For this review, take the finished solid that the model builds, in its own axes (mm). Face numbers are marked on the shaded views. A direction names the side the tool comes from. Round coordinates to 2 decimals unless told otherwise and drop trailing zeros. Loops run counter-clockwise (first coordinate to the right, second up) from the corner with the lowest first, then second, coordinate; pieces in that order, holes last.
1) Tool access review of the marked faces 1 and 2: name each direction out of +Z, -Z, +X, -X, +Y, -Y from which nothing blocks a thin tool from reaching the whole face with its end or side.
2) Wall thickness on L1, parallel to Z at x = 0, y = 0.3; L2, parallel to Y at x = 0, z = 50.7; L3, parallel to Y at x = 0, z = 51.45: over which ranges is each line inside the solid? List them lowest first.
3) Insertion check: pin 1 (4.5 mm diameter, centred on x = 0.5, z = 13.5, fed in from +Y); pin 2 (1 mm diameter, centred on x = 5.5, y = 45, fed in from -Z); pin 3 (4 mm diameter, centred on x = 0, z = 34.3, fed in from -Y). Each pin has a flat end and moves straight along its axis. Give the tip position at first contact, or say it passes through.
4) Take a section at B-B (x = 0). State the section outline as (y, z) points.
5) Take a section at D-D (x = 4.75). State the section outline as (y, z) points, then the cut area to 3 significant figures.
6) Take a section at A-A (y = 16.7). State the section outline as (x, z) points, then the cut area to 3 significant figures.
7) Take a section at C-C (z = 9.8). State the section outline as (x, y) points, then the cut area to 3 significant figures.
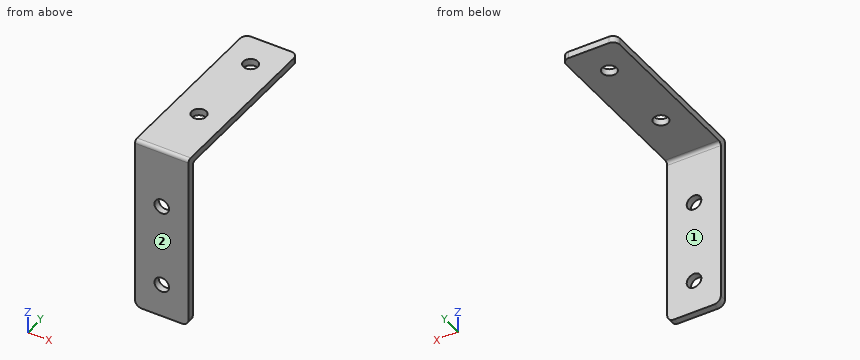
```python
from build123d import *

# Parameters (mm, degrees)
SKETCH_1_W          = 15.8
SKETCH_1_H          = 2
EXTRUDE_1_DEPTH     = 52
SKETCH_2_W          = 15.8
SKETCH_2_H          = 2
EXTRUDE_2_DEPTH     = 50
FILLET_5_R          = 1
FILLET_6_R          = 1
FILLET_7_R          = 2
FILLET_8_R          = 2
SKETCH_3_R          = 2.15
CUT_EXTRUDE_1_DEPTH = 50
SKETCH_8_R          = 2.15
CUT_EXTRUDE_3_DEPTH = 50


with BuildPart() as part:
    # 草圖1 → 填料-伸長1 (new body)
    with BuildSketch(Plane.XY):
        Rectangle(SKETCH_1_W, SKETCH_1_H)
    extrude(amount=EXTRUDE_1_DEPTH)

    # 草圖2 → 填料-伸長2 (add)
    with BuildSketch(Plane(origin=(0, 1, 0), x_dir=(1, 0, 0), z_dir=(0, 1, 0))):
        with Locations((0, -51)):
            Rectangle(SKETCH_2_W, SKETCH_2_H)
    extrude(amount=EXTRUDE_2_DEPTH)

    # 圓角5
    fillet_5_edges = [part.edges().sort_by_distance(p)[0] for p in [
        (0, -1, 52),
    ]]
    fillet(fillet_5_edges, radius=FILLET_5_R)

    # 圓角6
    fillet_6_edges = [part.edges().sort_by_distance(p)[0] for p in [
        (0, 1, 50),
    ]]
    fillet(fillet_6_edges, radius=FILLET_6_R)

    # 圓角7
    fillet_7_edges = [part.edges().sort_by_distance(p)[0] for p in [
        (7.9, 51, 51),
    ]]
    fillet(fillet_7_edges, radius=FILLET_7_R)

    # 圓角8
    fillet_8_edges = [part.edges().sort_by_distance(p)[0] for p in [
        (-7.9, 51, 51),
        (7.9, 0, 0),
        (-7.9, 0, 0),
    ]]
    fillet(fillet_8_edges, radius=FILLET_8_R)

    # 草圖3 → 除料-伸長1 (cut)
    with BuildSketch(Plane(origin=(0, 0, 50), x_dir=(-1, 0, 0), z_dir=(0, 0, -1))):
        with Locations((0, 41.2)):
            Circle(SKETCH_3_R)
        with Locations((0, 16.7)):
            Circle(SKETCH_3_R)
    extrude(amount=-CUT_EXTRUDE_1_DEPTH, mode=Mode.SUBTRACT)

    # 草圖8 → 除料-伸長3 (cut)
    with BuildSketch(Plane(origin=(0, 1, 0), x_dir=(1, 0, 0), z_dir=(0, 1, 0))):
        with Locations(Location((0, -9.8, 0), (0, 0, 180))):
            Circle(SKETCH_8_R)
        with Locations(Location((0, -34.3, 0), (0, 0, 180))):
            Circle(SKETCH_8_R)
    extrude(amount=-CUT_EXTRUDE_3_DEPTH, mode=Mode.SUBTRACT)


solid = part.part
```
Response:
1. face 1: -Z, +X, -X, +Y
1. face 2: +Z, -Z, +X, -X, -Y
2. L1: z = 0 to 7.65, 11.95 to 32.15, 36.45 to 52
2. L2: y = -1 to 14.55, 18.85 to 39.05, 43.35 to 51
2. L3: y = -0.89 to 14.55, 18.85 to 39.05, 43.35 to 51
3. pin 1: stops at y = 1
3. pin 2: stops at z = 50
3. pin 3: passes through
4. outline: (-1, 0) - (1, 0) - (1, 7.65) - (-1, 7.65) - close; (-1, 11.95) - (1, 11.95) - (1, 32.15) - (-1, 32.15) - close; (-1, 36.45) - (1, 36.45) - (1, 49) arc R1 cw to (2, 50) - (14.55, 50) - (14.55, 52) - (0, 52) arc R1 ccw to (-1, 51) - close; (18.85, 50) - (39.05, 50) - (39.05, 52) - (18.85, 52) - close; (43.35, 50) - (51, 50) - (51, 52) - (43.35, 52) - close
5. outline: (-1, 0) - (1, 0) - (1, 49) arc R1 cw to (2, 50) - (51, 50) - (51, 52) - (0, 52) arc R1 ccw to (-1, 51) - close
5. area: 204 mm2
6. outline: (-7.9, 50) - (-2.15, 50) - (-2.15, 52) - (-7.9, 52) - close; (2.15, 50) - (7.9, 50) - (7.9, 52) - (2.15, 52) - close
6. area: 23.0 mm2
7. outline: (-7.9, -1) - (-2.15, -1) - (-2.15, 1) - (-7.9, 1) - close; (2.15, -1) - (7.9, -1) - (7.9, 1) - (2.15, 1) - close
7. area: 23.0 mm2
